Design review of the part built by this model. Coordinates are the model's own, in mm. A direction names the side the tool comes from. Coordinates: 2 decimals unless noted, no trailing zeros. Write each loop counter-clockwise with the first axis right and the second up, starting at its lowest first coordinate (ties: lowest second). Pieces come first, ordered by that corner, then holes. Notation, with made-up numbers: (-32, -15.75) -> (14, -15.75) arc R22 cw to (14, 21.25) -> close; hole circle Ø4 at (67.25, 49.5). An arc over 180 degrees is marked (long way). Answer in a Markdown table with one row per item. Add a question column.
Item 1: Draft analysis for pull direction X (two halves, no side actions). For faces 1 (the face through (-3.048, 100.312, -0.017)), 2 (the face through (1.807, 100.312, 4.363)), 3 (the face through (5, 99.06, 0)), 4 (the face through (-1.79, 100.31, 4.32)), state which applies: released by +X, released by -X, zero draft, split by the parting line, or undercut.
Item 2: For faces 5 (the face through (3.048, 100.312, 0.017)), 6 (the face through (-4.363, 100.312, -1.807)), 7 (the face through (0, 99.06, -5)), 8 (the face through (-3, 101.6, 3)), 9 (the face through (0, 99.06, 5)), list the 3-axis set-ups (+Z, -Z, +X, -X, +Y, -Y) from which the entire face can be reached by the end or side of a thin tool; tool diameter is ignored.
Item 3: Clearance check with flat-ended pins moving along their axes: P1, Ø4, axis at y = 23, z = 4, coming from the -X side; P2, Ø1.2, axis at x = 6, y = 18.5, coming from the +Z side; P3, Ø0.5, axis at x = 6, y = 13, coming from the -Z side. State where each tip first meets the part, or that it passes through.
Item 4: Take a section at C-C, the plane y = 25.5. Write out the cut boundary in (x, z), and give its area (3 significant figures).
Item 5: To check wall thickness, follow line 1 (Z direction, x = 0, y = 96.75); line 2 (Y direction, x = 0.5, z = 4); line 3 (Z direction, x = -3.25, y = 39.5). State the ranges of each line that lie inside material, in increasing order.
Item 6: Take a section at A-A, the plane x = -4.5. Write out the cut boundary in (y, z), and give its area (3 significant figures).
Item 7: Take a section at B-B, the plane y = 75. Write out the cut boundary in (x, z).
from build123d import *

# Parameters (mm, degrees)
SKETCH1_R                        = 6.35
BOSS_EXTRUDE1_DEPTH              = 101.6
CUT_EXTRUDE1_DEPTH               = 40.64
FILLET1_R                        = 1.27
F_10_24_TAPPED_HOLE1_D           = 3.7973
F_10_24_TAPPED_HOLE1_DEPTH       = 12.954
F_10_24_TAPPED_HOLE1_CSINK_D     = 6.096
F_10_24_TAPPED_HOLE1_CSINK_ANGLE = 90
F_10_24_TAPPED_HOLE1_TIP         = 1.140824014
CUT_EXTRUDE3_START               = -2.54
CUT_EXTRUDE3_DEPTH               = 2.54


with BuildPart() as part:
    # Sketch1 → Boss-Extrude1 (new body)
    with BuildSketch(Plane(origin=(0, 0, 0), x_dir=(1, 0, 0), z_dir=(0, 1, 0))):
        with Locations(Location((0, 0, 0), (0, 0, 270))):
            Circle(SKETCH1_R)
    extrude(amount=BOSS_EXTRUDE1_DEPTH)

    # Sketch2 → Cut-Extrude1 (cut)
    with BuildSketch(Plane(origin=(0, 0, 0), x_dir=(-1, 0, 0), z_dir=(0, -1, 0))):
        with BuildLine():
            Line((-6.164407839, -1.524), (-5.08, -1.524))
            Line((-5.08, -1.524), (-5.08, 1.524))
            Line((-5.08, 1.524), (-6.164407839, 1.524))
            ThreePointArc((-6.164407839, 1.524), (-6.35, 0), (-6.164407839, -1.524))
        make_face()
    extrude(amount=-CUT_EXTRUDE1_DEPTH, mode=Mode.SUBTRACT)

    # Fillet1
    fillet1_edges = [part.edges().sort_by_distance(p)[0] for p in [
        (5.08, 40.64, 0),
    ]]
    fillet(fillet1_edges, radius=FILLET1_R - 0.0001)  # a hair under: the kernel refuses the full size

    # #10-24 Tapped Hole1
    with Locations(Plane(origin=(0, 101.6, 0), x_dir=(1, 0, 0), z_dir=(0, 1, 0))):
        with Locations((0, 0)):
            CounterSinkHole(F_10_24_TAPPED_HOLE1_D / 2, F_10_24_TAPPED_HOLE1_CSINK_D / 2, depth=F_10_24_TAPPED_HOLE1_DEPTH, counter_sink_angle=F_10_24_TAPPED_HOLE1_CSINK_ANGLE)
            with Locations((0, 0, -(F_10_24_TAPPED_HOLE1_DEPTH + F_10_24_TAPPED_HOLE1_TIP / 2))):  # 118° drill point
                Cone(0, F_10_24_TAPPED_HOLE1_D / 2, F_10_24_TAPPED_HOLE1_TIP, mode=Mode.SUBTRACT)

    # Sketch6 → Cut-Extrude3 (cut)
    with BuildSketch(Plane(origin=(0, 101.6, 0), x_dir=(1, 0, 0), z_dir=(0, 1, 0)).offset(CUT_EXTRUDE3_START)):
        with BuildLine():
            Line((2.430039796, -5.866635031), (1.166419102, -2.815984815))
            ThreePointArc((1.166419102, -2.815984815), (0, -3.048), (-1.166419102, -2.815984815))
            Line((-1.166419102, -2.815984815), (-2.430039796, -5.866635031))
            ThreePointArc((-2.430039796, -5.866635031), (0, -6.35), (2.430039796, -5.866635031))
        make_face()
        with BuildLine():
            Line((-5.866635031, 2.430039796), (-2.815984815, 1.166419102))
            ThreePointArc((-2.815984815, 1.166419102), (-3.048, 0), (-2.815984815, -1.166419102))
            Line((-2.815984815, -1.166419102), (-5.866635031, -2.430039796))
            ThreePointArc((-5.866635031, -2.430039796), (-6.35, 0), (-5.866635031, 2.430039796))
        make_face()
        with BuildLine():
            Line((2.430039796, 5.866635031), (1.166419102, 2.815984815))
            ThreePointArc((1.166419102, 2.815984815), (0, 3.048), (-1.166419102, 2.815984815))
            Line((-1.166419102, 2.815984815), (-2.430039796, 5.866635031))
            ThreePointArc((-2.430039796, 5.866635031), (0, 6.35), (2.430039796, 5.866635031))
        make_face()
        with BuildLine():
            Line((5.866635031, -2.430039796), (2.815984815, -1.166419102))
            ThreePointArc((2.815984815, -1.166419102), (3.048, 0), (2.815984815, 1.166419102))
            Line((2.815984815, 1.166419102), (5.866635031, 2.430039796))
            ThreePointArc((5.866635031, 2.430039796), (6.35, 0), (5.866635031, -2.430039796))
        make_face()
    extrude(amount=CUT_EXTRUDE3_DEPTH, mode=Mode.SUBTRACT)


solid = part.part
Answers:
| question | item | result |
|---|---|---|
| 1 | face 1 | released by -X |
| 1 | face 2 | undercut |
| 1 | face 3 | zero draft |
| 1 | face 4 | undercut |
| 2 | face 5 | +X, +Y |
| 2 | face 6 | -X, +Y |
| 2 | face 7 | -Z, +Y |
| 2 | face 8 | +Z, -Z, +X, -X, +Y |
| 2 | face 9 | +Z, +Y |
| 3 | P1 | stops at x = -6.03 |
| 3 | P2 | stops at z = 3.34 |
| 3 | P3 | stops at z = -2.69 |
| 4 | outline | (5.08, -1.52) -> (5.08, 1.52) -> (6.16, 1.52) arc R6.35 ccw (long way) to (6.16, -1.52) -> close |
| 4 | area | 123 mm^2 |
| 5 | line 1 | z = -6.35 to -1.9, 1.9 to 6.35 |
| 5 | line 2 | y = 0 to 99.06 |
| 5 | line 3 | z = -5.46 to 5.46 |
| 6 | outline | (0, -4.48) -> (101.6, -4.48) -> (101.6, -1.86) -> (99.06, -1.86) -> (99.06, 1.86) -> (101.6, 1.86) -> (101.6, 4.48) -> (0, 4.48) -> close |
| 6 | area | 901 mm^2 |
| 7 | outline | circle Ø12.7 at (0, 0) |
